from build123d import *

# Parameters (mm, degrees)
BOSS_EXTRUDE1_DEPTH      = 50.8
BOSS_EXTRUDE1_DEPTH_BACK = 12.7
SKETCH3_W                = 200.66
SKETCH3_H                = 143.51
SKETCH3_W_2              = 180.34
SKETCH3_H_2              = 123.19
SKETCH3_3_W              = 180.34
SKETCH3_3_H              = 123.19
BOSS_EXTRUDE2_DEPTH      = 12.7
BOSS_EXTRUDE3_DEPTH      = 63.5
CUT_EXTRUDE1_DEPTH       = 269.463806918
CUT_EXTRUDE1_DEPTH_BACK  = 269.463806918
SKETCH5_R                = 4.445
SKETCH5_R_2              = 1.000000032
SKETCH5_R_3              = 1
FILLET1_R                = 6.35
SKETCH7_W                = 88.9
SKETCH7_H                = 95.25
BOSS_EXTRUDE4_DEPTH      = 12.7
CHAMFER1_SIZE            = 21.336
CHAMFER2_START           = -163
CHAMFER2_OUTLINE_W       = 17
CHAMFER2_OUTLINE_H       = 17
CHAMFER2_DEPTH           = 6.818277269
CHAMFER3_START           = -193
CHAMFER3_OUTLINE_W       = 15
CHAMFER3_OUTLINE_H       = 17
CHAMFER3_DEPTH           = 6.465208093
CHAMFER4_SIZE            = 5.08
CHAMFER5_SIZE            = 5.08
FILLET3_R                = 10.16
CHAMFER6_SIZE            = 5.08
CUT_EXTRUDE2_DEPTH       = 299.446905332
CUT_EXTRUDE2_DEPTH_BACK  = 299.446905332
SKETCH8_R                = 10.16
SKETCH9_R                = 2
SKETCH9_R_2              = 2.000000064
CUT_EXTRUDE3_DEPTH       = 12.7


with BuildPart() as part:
    # Sketch3 → Boss-Extrude1 (new, two sides: drawn at the far end of the back side and taken through both)
    with BuildSketch(Plane(origin=(0, 0, 0), x_dir=(1, 0, 0), z_dir=(0, 1, 0)).offset(-BOSS_EXTRUDE1_DEPTH_BACK)):
        Rectangle(SKETCH3_W, SKETCH3_H)
        Rectangle(SKETCH3_W_2, SKETCH3_H_2, mode=Mode.SUBTRACT)
    extrude(amount=BOSS_EXTRUDE1_DEPTH + BOSS_EXTRUDE1_DEPTH_BACK)

    # Sketch3<3> → Boss-Extrude2 (add)
    with BuildSketch(Plane(origin=(0, 0, 0), x_dir=(1, 0, 0), z_dir=(0, 1, 0))):
        Rectangle(SKETCH3_3_W, SKETCH3_3_H)
    extrude(amount=-BOSS_EXTRUDE2_DEPTH)

    # Sketch4 → Boss-Extrude3 (add)
    with BuildSketch(Plane(origin=(0, -12.7, 0), x_dir=(-1, 0, 0), z_dir=(0, -1, 0))):
        Polygon((153.329999918, 56.515), (100.33, 56.515), (100.33, 40.005), (141.899999918, 40.005), (141.899999918, 19.685), (153.329999918, 19.685), align=None)
        Polygon((141.9, -40.005), (100.33, -40.005), (100.33, -56.515), (153.33, -56.515), (153.33, -19.685), (141.9, -19.685), align=None)
        Polygon((-100.33, 40.005), (-100.33, 56.515), (-153.329999918, 56.515), (-153.329999918, 19.685), (-141.899999918, 19.685), (-141.899999918, 40.005), align=None)
        Polygon((-100.33, -40.005), (-141.9, -40.005), (-141.9, -19.685), (-153.33, -19.685), (-153.33, -56.515), (-100.33, -56.515), align=None)
    extrude(amount=-BOSS_EXTRUDE3_DEPTH)

    # Sketch5 → Cut-Extrude1 (cut, two sides: drawn at the far end of the back side and taken through both)
    with BuildSketch(Plane.ZY.offset(100.33).offset(-CUT_EXTRUDE1_DEPTH_BACK)):
        with Locations(Location((0, 19.05, 0), (0, 0, 180))):
            Circle(SKETCH5_R)
        with Locations(Location((-9.017, 19.05, 0), (0, 0, 180))):
            Circle(SKETCH5_R_2)
        with Locations(Location((9.017, 19.05, 0), (0, 0, 180))):
            Circle(SKETCH5_R_3)
        with Locations(Location((0.017538483, 28.067, 0), (0, 0, 180))):
            Circle(SKETCH5_R_3)
        with Locations(Location((-0.055629344, 10.033, 0), (0, 0, 180))):
            Circle(SKETCH5_R_3)
    extrude(amount=CUT_EXTRUDE1_DEPTH + CUT_EXTRUDE1_DEPTH_BACK, mode=Mode.SUBTRACT)

    # Fillet1
    fillet1_edges = [part.edges().sort_by_distance(p)[0] for p in [
        (100.33, 19.05, -56.515),
        (100.33, 19.05, -40.005),
        (-100.33, 19.05, -40.005),
        (-100.33, 19.05, -56.515),
        (-100.33, 19.05, 40.005),
        (-100.33, 19.05, 56.515),
        (100.33, 19.05, 71.755),
        (-100.33, 19.05, 71.755),
        (100.33, 19.05, 56.515),
        (100.33, 19.05, 40.005),
    ]]
    fillet(fillet1_edges, radius=FILLET1_R)

    # Sketch7 → Boss-Extrude4 (add)
    with BuildSketch(Plane.ZY.offset(100.33)):
        with Locations((-116.205, 24.477736962)):
            Rectangle(SKETCH7_W, SKETCH7_H)
    extrude(amount=-BOSS_EXTRUDE4_DEPTH)

    # Chamfer1
    # the kernel refuses this chamfer: 21.336 mm, written as the material it takes off along each edge
    with BuildSketch(Plane(origin=(-155.199428231, 72.102736962, -71.755), x_dir=(0, -1, 0), z_dir=(1, 0, 0))) as chamfer1_piece_1_section:
        Polygon((CHAMFER1_SIZE, 0), (0, CHAMFER1_SIZE), (0, 0), align=None)
    chamfer1_piece_1 = extrude(amount=122.438856462, mode=Mode.PRIVATE)
    chamfer1_piece_1 = split(chamfer1_piece_1, bisect_by=Plane(origin=(-155.199428231, 50.8, -71.755), z_dir=(0, 1, 0)), keep=Keep.TOP, mode=Mode.PRIVATE)
    add(chamfer1_piece_1, mode=Mode.SUBTRACT)
    with BuildSketch(Plane(origin=(-155.199428231, -23.147263038, -71.755), x_dir=(0, 1, 0), z_dir=(1, 0, 0))) as chamfer1_piece_2_section:
        Polygon((CHAMFER1_SIZE, 0), (0, -CHAMFER1_SIZE), (0, 0), align=None)
    chamfer1_piece_2 = extrude(amount=122.438856462, mode=Mode.PRIVATE)
    chamfer1_piece_2 = split(chamfer1_piece_2, bisect_by=Plane(origin=(-155.199428231, -12.7, -71.755), z_dir=(0, -1, 0)), keep=Keep.TOP, mode=Mode.PRIVATE)
    add(chamfer1_piece_2, mode=Mode.SUBTRACT)

    # Chamfer2: read off the stored shape, not the designer's step
    # Chamfer2 outline → Chamfer2 (cut)
    with BuildSketch(Plane(origin=(0, 0, 0), x_dir=(0.8737038499063027, -0.34397789366389886, -0.34397789366389886), z_dir=(0.4864582023760161, 0.6178019170175401, 0.6178019170175401)).offset(CHAMFER2_START)):
        with Locations((-20.5, 97.5)):
            Rectangle(CHAMFER2_OUTLINE_W, CHAMFER2_OUTLINE_H)
    extrude(amount=CHAMFER2_DEPTH, mode=Mode.SUBTRACT)

    # Chamfer3: read off the stored shape, not the designer's step
    # Chamfer3 outline → Chamfer3 (cut)
    with BuildSketch(Plane(origin=(0, 0, 0), x_dir=(0.8164965809277258, 0.40824829046386313, -0.40824829046386313), z_dir=(0.5773502691896258, -0.5773502691896258, 0.5773502691896258)).offset(CHAMFER3_START)):
        with Locations((15.5, -62.5)):
            Rectangle(CHAMFER3_OUTLINE_W, CHAMFER3_OUTLINE_H)
    extrude(amount=CHAMFER3_DEPTH, mode=Mode.SUBTRACT)

    # Chamfer4
    chamfer4_edges = [part.edges().sort_by_distance(p)[0] for p in [
        (-90.17, 25.4, 61.595),
        (90.17, 25.4, 61.595),
    ]]
    chamfer(chamfer4_edges, length=CHAMFER4_SIZE)

    # Chamfer5
    chamfer5_edges = [part.edges().sort_by_distance(p)[0] for p in [
        (6.35, 50.8, -71.755),
    ]]
    chamfer(chamfer5_edges, length=CHAMFER5_SIZE)

    # Fillet3
    fillet3_edges = [part.edges().sort_by_distance(p)[0] for p in [
        (-87.63, 16.51, -71.755),
    ]]
    fillet(fillet3_edges, radius=FILLET3_R)

    # Chamfer6
    chamfer6_edges = [part.edges().sort_by_distance(p)[0] for p in [
        (-93.98, 72.102736962, -93.091),
    ]]
    chamfer(chamfer6_edges, length=CHAMFER6_SIZE)

    # Mirror1: part across plane


with BuildPart() as part_1:
    add(part.part)
    add(part.part.mirror(Plane.ZY))

    # Sketch8 → Cut-Extrude2 (cut, two sides: drawn at the far end of the back side and taken through both)
    with BuildSketch(Plane(origin=(-87.63, 0, 0), x_dir=(0, 0, -1), z_dir=(1, 0, 0)).offset(-CUT_EXTRUDE2_DEPTH_BACK)):
        with Locations((140.97, 34.002736962)):
            Circle(SKETCH8_R)
    extrude(amount=CUT_EXTRUDE2_DEPTH + CUT_EXTRUDE2_DEPTH_BACK, mode=Mode.SUBTRACT)

    # Sketch9 → Cut-Extrude3 (cut)
    with BuildSketch(Plane(origin=(0, 50.8, 0), x_dir=(1, 0, 0), z_dir=(0, 1, 0))):
        with Locations(Location((-94.488, 65.948922821, 0), (0, 0, 270))):
            Circle(SKETCH9_R)
        with Locations(Location((-95.25, 32.385, 0), (0, 0, 270))):
            Circle(SKETCH9_R)
        with Locations(Location((-94.361, -62.865, 0), (0, 0, 270))):
            Circle(SKETCH9_R_2)
        with Locations(Location((92.71, -62.865, 0), (0, 0, 270))):
            Circle(SKETCH9_R)
        with Locations(Location((92.71, 66.675, 0), (0, 0, 270))):
            Circle(SKETCH9_R)
        with Locations(Location((95.25, 32.385, 0), (0, 0, 270))):
            Circle(SKETCH9_R)
    extrude(amount=-CUT_EXTRUDE3_DEPTH, mode=Mode.SUBTRACT)


solid = part_1.part
Here's how the part is built. I have some questions about the finished solid (model axes, mm). A direction names the side the tool comes from. Give positions to 0.01 mm unless a question says otherwise; leave off trailing zeros. Loops run counter-clockwise (first coordinate to the right, second up) from the corner with the lowest first, then second, coordinate; pieces in that order, holes last. Notation, with made-up numbers: (-21.75, -36.5) -> (-8.75, -36.5) arc R9 cw to (-8.75, -31.5) -> close; hole circle Ø6 at (-18.75, 48). An arc over 180 degrees is marked (long way). Answer as a JSON object with one key per item and string values. Group by question number.
Item 1: Imagine slicing it at C-C on x = -68. Write out the boundary of the cut face in (y, z) (3 decimals), then the cut area to 3 significant figures.
Item 2: Imagine slicing it at A-A on z = -140.97. Write out the boundary of the cut face in (x, y).
Item 3: Will these pins go through, and if not, where does the flat tip stop? pin 1 (9 mm diameter, centred on x = -145, y = 16, fed in from -Z) (3 decimals); pin 2 (4 mm diameter, centred on x = 99.5, z = -79.5, fed in from +Y); pin 3 (1.2 mm diameter, centred on y = 19.05, z = -9.017, fed in from -X); pin 4 (1.5 mm diameter, centred on x = -118.5, y = 23, fed in from +Z) (3 decimals).
Item 4: Thinking about a two-plate mould opening in Z: for faces 4 (the flat face through (-100.33, 25, -112)), 5 (the flat face through (90.17, 25, -2)), 6 (the flat face through (-95, -20, -158)), which applies, pulls with the +Z half, pulls with the -Z half, needs draft (parallel to the pull), parting line crosses it, or undercut?
Item 5: I need wall thicknesses on L1, parallel to X at y = 44.5, z = -25.5; L2, parallel to Z at x = 93, y = 19 (3 decimals); L3, parallel to Z at x = -75, y = 12.5 (3 decimals). Which ranges of each line are inside material? Lowest first, please.
Item 6: On a 3-axis mill with a long thin cutter (end or side, diameter ignored), from which of +Z, -Z, +X, -X, +Y, -Y can I reach the whole of each face in a straight line? I mean faces 1 (the flat face through (-125, 19, 40.005)), 2 (the flat face through (-1, 25, -61.595)), 3 (the flat face through (148, 19, -19.685)). Say none if no direction works.
Item 7: Imagine slicing it at B-B on x = 133.5. Write out the boundary of the cut face in (y, z) (3 decimals), then the cut area to 3 significant figures.
Answer list:
{
 "1": {"outline": "(-12.7, -71.755) -> (45.72, -71.755) -> (50.8, -66.675) -> (50.8, -61.595) -> (0, -61.595) -> (0, 61.595) -> (50.8, 61.595) -> (50.8, 71.755) -> (-12.7, 71.755) -> close", "area": "2,840 mm2"},
 "2": {"outline": "(-100.33, -23.15) -> (-87.63, -23.15) -> (-87.63, 23.84) -> (-100.33, 23.84) -> close; (-100.33, 44.16) -> (-87.63, 44.16) -> (-87.63, 72.1) -> (-100.33, 72.1) -> close; (87.63, -23.15) -> (100.33, -23.15) -> (100.33, 23.84) -> (87.63, 23.84) -> close; (87.63, 44.16) -> (100.33, 44.16) -> (100.33, 72.1) -> (87.63, 72.1) -> close"},
 "3": {"pin 1": "stops at z = -56.515", "pin 2": "stops at y = 60.51", "pin 3": "passes through", "pin 4": "stops at z = 56.515"},
 "4": {"face 4": "needs draft", "face 5": "undercut", "face 6": "pulls with the -Z half"},
 "5": {"L1": "x = -153.33 to -141.9, -100.33 to -90.17, 90.17 to 100.33, 141.9 to 153.33", "L2": "z = -160.655 to -10.016, -8.018 to -4.445, 4.445 to 8.018, 10.016 to 71.755", "L3": "z = -71.755 to -61.595, 61.595 to 71.755"},
 "6": {"face 1": "+Y, -Y", "face 2": "+Y", "face 3": "+X, +Y, -Y"},
 "7": {"outline": "(-12.7, -56.515) -> (50.8, -56.515) -> (50.8, -40.005) -> (-12.7, -40.005) -> close; (-12.7, 40.005) -> (50.8, 40.005) -> (50.8, 56.515) -> (-12.7, 56.515) -> close", "area": "2,100 mm2"}
}
